```python
from build123d import *

# Parameters (mm, degrees)
ESQUISSE3_W      = 400
ESQUISSE3_H      = 40
EXTRUSION1_DEPTH = 110
ESQUISSE8_W      = 400
ESQUISSE8_H      = 122
EXTRUSION3_DEPTH = 15
ESQUISSE11_W     = 400
ESQUISSE11_H     = 110
EXTRUSION5_DEPTH = 6
ESQUISSE10_R     = 3
EXTRUSION4_DEPTH = 1.5
ESQUISSE12_R     = 3
EXTRUSION6_DEPTH = 20


with BuildPart() as part:
    # Esquisse3 → Extrusion1 (new body)
    with BuildSketch(Plane.XY):
        with Locations((38, 5)):
            Rectangle(ESQUISSE3_W, ESQUISSE3_H)
    extrude(amount=EXTRUSION1_DEPTH)

    # Esquisse8 → Extrusion3 (add)
    with BuildSketch(Plane(origin=(0, 25, 0), x_dir=(1, 0, 0), z_dir=(0, 1, 0))):
        with Locations((38, -49)):
            Rectangle(ESQUISSE8_W, ESQUISSE8_H)
    extrude(amount=EXTRUSION3_DEPTH)

    # Esquisse11 → Extrusion5 (add)
    with BuildSketch(Plane.XZ.offset(15)):
        with Locations((38, 55)):
            Rectangle(ESQUISSE11_W, ESQUISSE11_H)
    extrude(amount=EXTRUSION5_DEPTH)

    # Esquisse10 → Extrusion4 (cut)
    with BuildSketch(Plane(origin=(0, 0, 0), x_dir=(-1, 0, 0), z_dir=(0, 0, -1))):
        with BuildLine():
            Line((59.5, -8), (59.5, -19))
            ThreePointArc((59.5, -19), (58.914213562, -20.414213562), (57.5, -21))
            Line((57.5, -21), (-68.5, -21))
            ThreePointArc((-68.5, -21), (-69.914213562, -20.414213562), (-70.5, -19))
            Line((-70.5, -19), (-70.5, -8))
            ThreePointArc((-70.5, -8), (-71.085786438, -6.585786438), (-72.5, -6))
            Line((-72.5, -6), (-83, -6))
            ThreePointArc((-83, -6), (-95.5, 6.5), (-83, 19))
            Line((-83, 19), (70.25, 19))
            ThreePointArc((70.25, 19), (82.75, 6.5), (70.25, -6))
            Line((70.25, -6), (61.5, -6))
            ThreePointArc((61.5, -6), (60.085786438, -6.585786438), (59.5, -8))
        make_face()
        with Locations((-86.5, 6.5)):
            Circle(ESQUISSE10_R, mode=Mode.SUBTRACT)
        with Locations((-20.5, 6.5)):
            Circle(ESQUISSE10_R, mode=Mode.SUBTRACT)
        with Locations((72.75, 6.5)):
            Circle(ESQUISSE10_R, mode=Mode.SUBTRACT)
        with BuildLine():
            Line((-31.5, -3), (-61.5, -3))
            ThreePointArc((-61.5, -3), (-62.207106781, -2.707106781), (-62.5, -2))
            Line((-62.5, -2), (-62.5, 12))
            ThreePointArc((-62.5, 12), (-62.207106781, 12.707106781), (-61.5, 13))
            Line((-61.5, 13), (-31.5, 13))
            ThreePointArc((-31.5, 13), (-30.792893219, 12.707106781), (-30.5, 12))
            Line((-30.5, 12), (-30.5, -2))
            ThreePointArc((-30.5, -2), (-30.792893219, -2.707106781), (-31.5, -3))
        make_face(mode=Mode.SUBTRACT)
        with BuildLine():
            Line((51.75, 0), (12.75, 0))
            ThreePointArc((12.75, 0), (12.042893219, 0.292893219), (11.75, 1))
            Line((11.75, 1), (11.75, 11))
            ThreePointArc((11.75, 11), (12.042893219, 11.707106781), (12.75, 12))
            Line((12.75, 12), (51.75, 12))
            ThreePointArc((51.75, 12), (52.457106781, 11.707106781), (52.75, 11))
            Line((52.75, 11), (52.75, 1))
            ThreePointArc((52.75, 1), (52.457106781, 0.292893219), (51.75, 0))
        make_face(mode=Mode.SUBTRACT)
    extrude(amount=-EXTRUSION4_DEPTH, mode=Mode.SUBTRACT)

    # Esquisse12 → Extrusion6 (cut)
    with BuildSketch(Plane(origin=(0, 0, 0), x_dir=(-1, 0, 0), z_dir=(0, 0, -1))):
        with Locations((-86.5, 6.5)):
            Circle(ESQUISSE12_R)
        with Locations((-20.5, 6.5)):
            Circle(ESQUISSE12_R)
        with Locations((72.75, 6.5)):
            Circle(ESQUISSE12_R)
        with BuildLine():
            Line((-30.5, -2), (-30.5, 12))
            ThreePointArc((-30.5, 12), (-30.792893219, 12.707106781), (-31.5, 13))
            Line((-31.5, 13), (-61.5, 13))
            ThreePointArc((-61.5, 13), (-62.207106781, 12.707106781), (-62.5, 12))
            Line((-62.5, 12), (-62.5, -2))
            ThreePointArc((-62.5, -2), (-62.207106781, -2.707106781), (-61.5, -3))
            Line((-61.5, -3), (-31.5, -3))
            ThreePointArc((-31.5, -3), (-30.792893219, -2.707106781), (-30.5, -2))
        make_face()
        with BuildLine():
            Line((52.75, 1), (52.75, 11))
            ThreePointArc((52.75, 11), (52.457106781, 11.707106781), (51.75, 12))
            Line((51.75, 12), (12.75, 12))
            ThreePointArc((12.75, 12), (12.042893219, 11.707106781), (11.75, 11))
            Line((11.75, 11), (11.75, 1))
            ThreePointArc((11.75, 1), (12.042893219, 0.292893219), (12.75, 0))
            Line((12.75, 0), (51.75, 0))
            ThreePointArc((51.75, 0), (52.457106781, 0.292893219), (52.75, 1))
        make_face()
    extrude(amount=-EXTRUSION6_DEPTH, mode=Mode.SUBTRACT)


solid = part.part
```
Model file for the job. Use its own axes, mm. A direction names the side the tool comes from. Coordinates: 2 decimals unless noted, no trailing zeros. Order: outer loops, then holes, each group sorted by start corner. A loop starts at its lowest first (then second) coordinate and runs counter-clockwise, first axis right, second up. Notation, with made-up numbers: (-27, 83.25) -> (-22, 83.25) arc R18 ccw to (-22, 96.25) -> close; hole circle Ø11 at (59.25, 73). An arc over 180 degrees is marked (long way). Return JSON: item names as keys, results as strings.
Item 1: 3-axis set-ups, long thin cutter, end or side, ignore diameter. For faces 4 (the face through (35, 40, 48)), 5 (the face through (35, 25, -6)), 6 (the face through (-32, 6, 20)): which of +Z, -Z, +X, -X, +Y, -Y reach the whole face in a straight line?
Model answer:
{"face 4": "+Z, -Z, +X, -X, +Y", "face 5": "-Z, +X, -X, -Y", "face 6": "-Z"}
Item 2: Pin check, flat tips, straight feed: P1, Ø5, axis at x = 133, y = -3, coming from the -Z side; P2, Ø5.5, axis at x = -72.75, y = 6.5, coming from the -Z side; P3, Ø5, axis at x = 21, y = 7.5, coming from the -Z side. Stop position of each tip, or through.
Model answer:
{"P1": "stops at z = 0", "P2": "stops at z = 20", "P3": "stops at z = 1.5"}
Item 3: Mould opens along X. For faces 1 (the face through (35, -21, 56)), 2 (the face through (-162, 10, 48)), 3 (the face through (30.5, 5, 11)) say: pulls with the +X half, pulls with the -X half, needs draft (parallel to the pull), parting line crosses it, or undercut.
Model answer:
{"face 1": "needs draft", "face 2": "pulls with the -X half", "face 3": "undercut"}
Item 4: Wall check: line 1 along X through (y, z) = (6, 13); line 2 along Y through (x, z) = (-72.75, 9.75); line 3 along Z through (x, y) = (-51.5, 17). Give the ranges that are in metal, low to high. Write a range as from..to.
Model answer:
{"line 1": "x = -162..-75.71, -69.79..-52.75, -11.75..17.54, 23.46..30.5, 62.5..83.54, 89.46..238", "line 2": "y = -21..3.5, 9.5..40", "line 3": "z = 1.5..110"}
Item 5: Slice it at A-A (x = -109). Write the cut outline in (y, z).
Model answer:
{"outline": "(-21, 0) -> (25, 0) -> (25, -12) -> (40, -12) -> (40, 110) -> (-21, 110) -> close"}
